Part print with two shaded views. Sizes in mm from the minimum x, y, z corner. A direction names the side the tool comes from. Coordinates: 2 decimals unless noted, no trailing zeros. Loops run counter-clockwise (first coordinate to the right, second up) from the corner with the lowest first, then second, coordinate; pieces in that order, holes last.
Item 1: Cut at C-C (x = 18). List the corners of the cut face in (y, z), and give its area (3 significant figures).
Item 2: 3-axis set-ups, long thin cutter, end or side, ignore diameter. For the marked faces 1, 2, 3 and 4: which of +Z, -Z, +X, -X, +Y, -Y reach the whole face in a straight line?
Item 3: Cut at B-B (z = 29.5). List the corners of the cut face in (x, y).
Item 4: Flat gauge pins, fed straight in: pin 1 (5 mm diameter, centred on y = 31, z = 27, fed in from +X); pin 2 (13.5 mm diameter, centred on x = 68.5, z = 25.5, fed in from +Y); pin 3 (1 mm diameter, centred on x = 60.5, z = 41.5, fed in from +Y). Where does each tip first touch, or does it go through?
Item 5: Cut at D-D (z = 37). List the corners of the cut face in (x, y).
Item 6: Cut at A-A (x = 42). List the corners of the cut face in (y, z) (3 decimals), and give its area (3 significant figures).
Item 7: Drill centre lines: line 1 along X through (y, z) = (33, 7); line 2 along Z through (x, y) = (69, 17.5); line 3 along Y through (x, z) = (37, 14). Where is each one in solid material? Low to high.
Item 8: Mould opens along Z. For the marked faces 5, 6 and 7 say: released by +Z, released by -Z, zero draft, split by the parting line, or undercut.
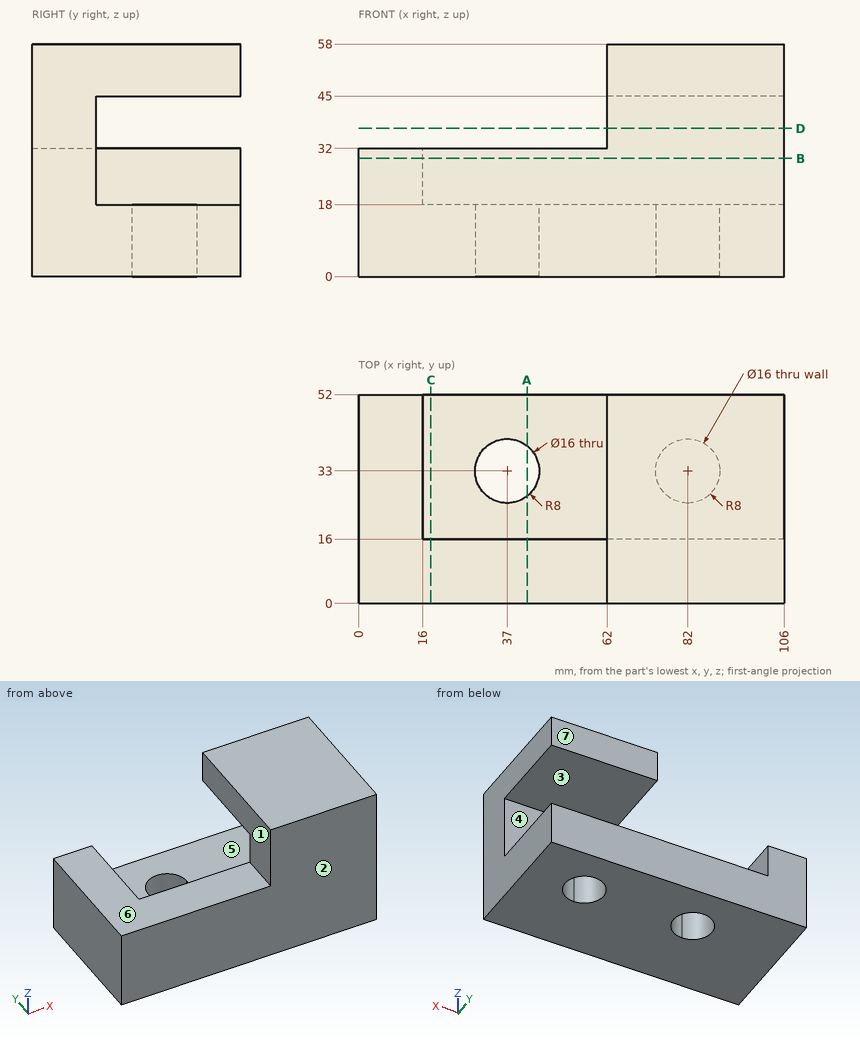
Filled sheet:
1. outline: (0, 0) - (52, 0) - (52, 18) - (16, 18) - (16, 32) - (0, 32) - close
1. area: 1,160 mm2
2. face 1: +Z, -X, +Y, -Y
2. face 2: +Z, -Z, +X, -X, -Y
2. face 3: +X, -X, +Y
2. face 4: +X, +Y
3. outline: (0, 0) - (106, 0) - (106, 16) - (16, 16) - (16, 52) - (0, 52) - close
4. pin 1: stops at x = 16
4. pin 2: stops at y = 16
4. pin 3: passes through
5. outline: (62, 0) - (106, 0) - (106, 16) - (62, 16) - close
6. outline: (0, 0) - (26.755, 0) - (26.755, 18) - (16, 18) - (16, 32) - (0, 32) - close; (39.245, 0) - (52, 0) - (52, 18) - (39.245, 18) - close
6. area: 935 mm2
7. line 1: x = 0 to 29, 45 to 74, 90 to 106
7. line 2: z = 0 to 18, 45 to 58
7. line 3: y = 0 to 25, 41 to 52
8. face 5: undercut
8. face 6: released by +Z
8. face 7: zero draft
